Geometry check sheet. Reference: the model listing, model coordinates, mm. A direction names the side the tool comes from. Round coordinates to 2 decimals unless told otherwise and drop trailing zeros. Loops run counter-clockwise (first coordinate to the right, second up) from the corner with the lowest first, then second, coordinate; pieces in that order, holes last. Notation, with made-up numbers: (26, 12) -> (76, 12) arc R32 cw to (76, 43) -> close; hole circle Ø9 at (48.25, 88.25). An arc over 180 degrees is marked (long way). Use a Markdown table: item, result. Add a question column.
Q1. Gauge pin test, flat ends, axial feed: P1, Ø5, axis at y = 4, z = 24.5, coming from the +X side; P2, Ø2, axis at y = 20, z = 4.5, coming from the +X side; P3, Ø3, axis at x = -21, z = -9.5, coming from the -Y side; P4, Ø7.5, axis at x = 44, y = 15, coming from the -Z side. Record the tip position at first contact, or that the pin passes through.
Q2. Sectioned sample at B-B, the plane z = 0. Give the number of separate pieces and of enclosed holes in the cut face, then the cut area to 3 significant figures.
Q3. Sectioned sample at D-D, the plane z = -15. Enter the section's corners in (x, y), then the cut area to 3 significant figures.
Q4. Material ranges on L1, parallel to Z at x = 39, y = 7.25; L2, parallel to X at y = 11.75, z = 0; L3, parallel to Y at x = 11, z = 11, recorded low to high.
Q5. Sectioned sample at A-A, the plane x = -25. Enter the section's corners in (y, z), then the cut area to 3 significant figures.
Q6. Set-up check for faces 4 (the face through (0.49, 18.1, -32.14)), 5 (the face through (-23, 6, 1)), 6 (the face through (46, 14, 30)), 7 (the face through (14, 20.5, -0.9)): record each of +Z, -Z, +X, -X, +Y, -Y from which the full face is reachable in a straight line by a thin tool's end or side.
Q7. Release check for a two-part mould opening along X. For faces 1 (the face through (48, 3, 34)), 2 (the face through (0, 21, 0)), 3 (the face through (-21, 20.5, -0.9)) record: released by +X, released by -X, zero draft, split by the parting line, or undercut.
```python
from build123d import *

# Parameters (mm, degrees)
SKETCH1_W                                     = 100
SKETCH1_H                                     = 70
BOSS_EXTRUDE1_DEPTH                           = 21
FILLET1_R                                     = 15
FILLET2_R                                     = 5
SHELL1_T                                      = -2
SKETCH2_W                                     = 34.075485645
SKETCH2_H                                     = 60
CUT_EXTRUDE1_DEPTH                            = 45
BOSS_EXTRUDE2_REACH                           = 64.849
SKETCH4_R                                     = 3
BOSS_EXTRUDE2_DRAFT                           = -5
CSK_FOR_M10_FLAT_HEAD_MACHINE_SCREW4_AT_COUNT = 2
CSK_FOR_M10_FLAT_HEAD_MACHINE_SCREW4_AT_PITCH = 35


with BuildPart() as part:
    # Sketch1 → Boss-Extrude1 (new body)
    with BuildSketch(Plane(origin=(0, 0, 0), x_dir=(1, 0, 0), z_dir=(0, 1, 0))):
        Rectangle(SKETCH1_W, SKETCH1_H)
    extrude(amount=BOSS_EXTRUDE1_DEPTH)

    # Fillet1
    fillet1_edges = [part.edges().sort_by_distance(p)[0] for p in [
        (-50, 21, 0),
        (50, 21, 0),
    ]]
    fillet(fillet1_edges, radius=FILLET1_R)

    # Fillet2
    fillet2_edges = [part.edges().sort_by_distance(p)[0] for p in [
        (0, 21, -35),
        (0, 21, 35),
        (-50, 3, -35),
        (50, 3, -35),
        (-45.606601718, 16.606601718, -35),
        (45.606601718, 16.606601718, -35),
        (50, 3, 35),
        (-50, 3, 35),
        (-45.606601718, 16.606601718, 35),
        (45.606601718, 16.606601718, 35),
    ]]
    fillet(fillet2_edges, radius=FILLET2_R)

    # Shell1
    shell1_openings = [part.faces().sort_by_distance(p)[0] for p in [
        (0, 0, 0),
    ]]
    offset(amount=SHELL1_T, openings=shell1_openings, kind=Kind.INTERSECTION)

    # Sketch2 → Cut-Extrude1 (cut)
    with BuildSketch(Plane(origin=(0, 21, 0), x_dir=(1, 0, 0), z_dir=(0, 1, 0))):
        with Locations((52.037742823, 0)):
            Rectangle(SKETCH2_W, SKETCH2_H)
    extrude(amount=-CUT_EXTRUDE1_DEPTH, mode=Mode.SUBTRACT)




with BuildPart() as boss_extrude2_long_prism_1:
    # Sketch4 → Boss-Extrude2 (the long prism of profile 1, to be tilted and cut off)
    with BuildSketch(Plane(origin=(0, 6, 0), x_dir=(1, 0, 0), z_dir=(0, 1, 0))):
        with Locations((-25, 0)):
            Circle(SKETCH4_R)
    extrude(amount=BOSS_EXTRUDE2_REACH)
    boss_extrude2_tool1_sides = [boss_extrude2_long_prism_1.faces().sort_by_distance(p)[0] for p in [
        (-28, 38.4245, 0),
    ]]
    draft(boss_extrude2_tool1_sides, Plane(origin=(0, 6, 0), x_dir=(1, 0, 0), z_dir=(0, 1, 0)), BOSS_EXTRUDE2_DRAFT)  # the draft: side faces tilted about the start plane


with BuildPart() as part_1:
    add(part.part)
    boss_extrude2_tool1 = boss_extrude2_long_prism_1.part - part.part



with BuildPart() as boss_extrude2_long_prism_2:
    # Sketch4 → Boss-Extrude2 (the long prism of profile 2, to be tilted and cut off)
    with BuildSketch(Plane(origin=(0, 6, 0), x_dir=(1, 0, 0), z_dir=(0, 1, 0))):
        with Locations((10, 0)):
            Circle(SKETCH4_R)
    extrude(amount=BOSS_EXTRUDE2_REACH)
    boss_extrude2_tool2_sides = [boss_extrude2_long_prism_2.faces().sort_by_distance(p)[0] for p in [
        (7, 38.4245, 0),
    ]]
    draft(boss_extrude2_tool2_sides, Plane(origin=(0, 6, 0), x_dir=(1, 0, 0), z_dir=(0, 1, 0)), BOSS_EXTRUDE2_DRAFT)  # the draft: side faces tilted about the start plane


with BuildPart() as part_2:
    add(part_1.part)
    boss_extrude2_tool2 = boss_extrude2_long_prism_2.part - part.part
    add(boss_extrude2_tool1.solids().sort_by_distance((-25, 6, 0))[0])
    add(boss_extrude2_tool2.solids().sort_by_distance((10, 6, 0))[0])

    # Sketch13 → CSK for M10 Flat Head Machine Screw4 (revolve, cut)
    with BuildSketch(Plane(origin=(-25, 21, 0), x_dir=(0, 0, 1), z_dir=(1, 0, 0))):
        Polygon((0, 0), (0, 15), (1.95, 15), (1.95, 3.15), (4.1, 1), (4.1, 0), align=None)
    csk_for_m10_flat_head_machine_screw4 = revolve(axis=Axis((-25, 27.35, 0), (0, -1, 0)), mode=Mode.SUBTRACT)

    # CSK for M10 Flat Head Machine Screw4 at: CSK for M10 Flat Head Machine Screw4 ×2
    with Locations(*[(i * CSK_FOR_M10_FLAT_HEAD_MACHINE_SCREW4_AT_PITCH, 0, 0) for i in range(1, CSK_FOR_M10_FLAT_HEAD_MACHINE_SCREW4_AT_COUNT)]):
        add(csk_for_m10_flat_head_machine_screw4, mode=Mode.SUBTRACT)


solid = part_2.part
```
Values:
| question | item | result |
|---|---|---|
| 1 | P1 | x = -47.99 |
| 1 | P2 | x = 35 |
| 1 | P3 | y = 19 |
| 1 | P4 | z = -35 |
| 2 | separate pieces | 3 |
| 2 | enclosed holes | 0 |
| 2 | area | 247 mm^2 |
| 3 | outline | (-50, 0) -> (-48, 0) -> (-48, 6) arc R13 cw to (-35, 19) -> (35, 19) -> (35, 21) -> (-35, 21) arc R15 ccw to (-50, 6) -> close |
| 3 | area | 196 mm^2 |
| 4 | L1 | -35 to -33, 33 to 35 |
| 4 | L2 | -48.85 to -46.66, -28.5 to -26.95, -23.05 to -21.5, 6.5 to 8.05, 11.95 to 13.5 |
| 4 | L3 | 19 to 21 |
| 5 | outline | (0, -35) -> (16, -35) arc R5 ccw to (21, -30) -> (21, -4.1) -> (20, -4.1) -> (17.85, -1.95) -> (6, -1.95) -> (6, -3) -> (19, -4.14) -> (19, -30) arc R3 cw to (16, -33) -> (0, -33) -> close; (0, 33) -> (16, 33) arc R3 cw to (19, 30) -> (19, 4.14) -> (6, 3) -> (6, 1.95) -> (17.85, 1.95) -> (20, 4.1) -> (21, 4.1) -> (21, 30) arc R5 ccw to (16, 35) -> (0, 35) -> close |
| 5 | area | 234 mm^2 |
| 6 | face 4 | -Y |
| 6 | face 5 | +X, -Y |
| 6 | face 6 | +X, +Y, -Y |
| 6 | face 7 | +Y |
| 7 | face 1 | released by +X |
| 7 | face 2 | zero draft |
| 7 | face 3 | undercut |
